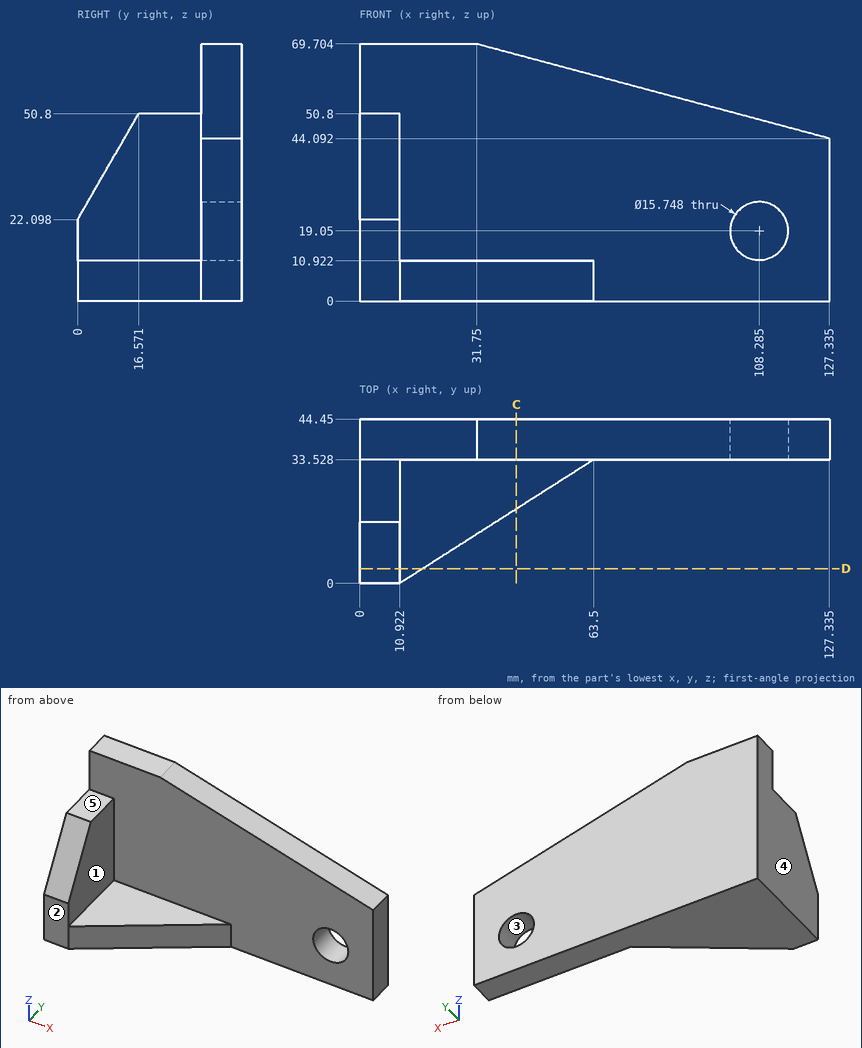
The figure shows three views and two pictorial views of one solid part (mm, origin at its lowest corner). Answer the questions. A direction names the side the tool comes from. Coordinates: 2 decimals unless noted, no trailing zeros. Order: outer loops, then holes, each group sorted by start corner. A loop starts at its lowest first (then second) coordinate and runs counter-clockwise, first axis right, second up.
Q1. Given P1, Ø10, axis at y = 14, z = 40.5, coming from the +X side; P2, Ø5, axis at x = 52, z = 24, coming from the -Y side; P3, Ø8.5, axis at x = 6, y = 24.5, coming from the +Z side, each flat-ended and moving along its own axis, determine where each tip first touches the part or whether it passes through.
Q2. For a pull along X with two mould halves and no side action, classify the marked faces 3, 4 and 5 as pulls with the +X half, pulls with the -X half, needs draft (parallel to the pull), parting line crosses it, or undercut.
Q3. Consider line 1 (X direction, y = 40, z = 19) (1 decimal); line 2 (Y direction, x = 110, z = 29.5); line 3 (Z direction, x = 12, y = 19). Determine where each line is inside the solid, lowest interval first.
Q4. A cutting plane is placed at C-C, the plane x = 42.5. Write down the section's boundary in (y, z).
Q5. Which of the six approach directions +Z, -Z, +X, -X, +Y, -Y give full straight-line access (tool end or side, diameter ignored) to the marked faces 1 and 2?
Q6. A cutting plane is placed at D-D, the plane y = 4. Write down the section's boundary in (x, z) (1 decimal).
Answers follow:
1. P1: stops at x = 10.92
1. P2: stops at y = 33.53
1. P3: stops at z = 50.8
2. face 3: undercut
2. face 4: pulls with the -X half
2. face 5: needs draft
3. line 1: x = 0 to 100.4, 116.2 to 127.3
3. line 2: y = 33.53 to 44.45
3. line 3: z = 0 to 10.92
4. outline: (20.14, 0) - (44.45, 0) - (44.45, 66.82) - (33.53, 66.82) - (33.53, 10.92) - (20.14, 10.92) - close
5. face 1: +Z, +X, -Y
5. face 2: +Z, -Z, +X, -X, -Y
6. outline: (0, 0) - (17.2, 0) - (17.2, 10.9) - (10.9, 10.9) - (10.9, 29) - (0, 29) - close
